The listing builds one solid part. Answer for the finished solid, in the listing's coordinates (mm). A direction names the side the tool comes from. Coordinates: 2 decimals unless noted, no trailing zeros. Order: outer loops, then holes, each group sorted by start corner. A loop starts at its lowest first (then second) coordinate and runs counter-clockwise, first axis right, second up. Notation, with made-up numbers: (-37.5, 12.25) -> (18.5, 12.25) arc R10 ccw to (18.5, 21.25) -> close; hole circle Ø2 at (-21.5, 35.25). An arc over 180 degrees is marked (long way). Return JSON: item names as keys, results as strings.
```python
from build123d import *

# Parameters (mm, degrees)
EXTRUDE_1_DEPTH     = 8.5
SKETCH_2_R          = 1.7
CUT_EXTRUDE_1_DEPTH = 34.737960816


with BuildPart() as part:
    # 草图1 → 凸台-拉伸1 (new body)
    with BuildSketch(Plane(origin=(0, 0, 0), x_dir=(1, 0, 0), z_dir=(0, 1, 0))):
        with BuildLine():
            Line((-25, -21), (25, -21))
            Line((25, -21), (25, -9))
            Line((25, -9), (11.788272368, -9))
            Line((11.788272368, -9), (6.375, -11.899973739))
            ThreePointArc((6.375, -11.899973739), (0, -13.5), (-6.375, -11.899973739))
            Line((-6.375, -11.899973739), (-11.788272368, -9))
            Line((-11.788272368, -9), (-25, -9))
            Line((-25, -9), (-25, -21))
        make_face()
    extrude(amount=EXTRUDE_1_DEPTH)

    # 草图2 → 切除-拉伸1 (cut, through all)
    with BuildSketch(Plane(origin=(0, 8.5, 0), x_dir=(1, 0, 0), z_dir=(0, 1, 0))):
        with Locations(Location((6, -17, 0), (0, 0, 270))):
            Circle(SKETCH_2_R)
        with Locations(Location((-6, -17, 0), (0, 0, 90))):
            Circle(SKETCH_2_R)
    extrude(amount=-CUT_EXTRUDE_1_DEPTH, mode=Mode.SUBTRACT)


solid = part.part
```
Item 1: The part is cut by section A-A on z = 17. Determine the outline of the cut face in (x, y), plus the area to 3 significant figures.
Answer list:
{"outline": "(-25, 0) -> (-7.7, 0) -> (-7.7, 8.5) -> (-25, 8.5) -> close; (-4.3, 0) -> (4.3, 0) -> (4.3, 8.5) -> (-4.3, 8.5) -> close; (7.7, 0) -> (25, 0) -> (25, 8.5) -> (7.7, 8.5) -> close", "area": "367 mm2"}
Item 2: The part is cut by section D-D on z = 10. Determine the outline of the cut face in (x, y).
Answer list:
{"outline": "(-25, 0) -> (-9.92, 0) -> (-9.92, 8.5) -> (-25, 8.5) -> close; (9.92, 0) -> (25, 0) -> (25, 8.5) -> (9.92, 8.5) -> close"}
Item 3: The part is cut by section C-C on x = 5.5. Determine the outline of the cut face in (y, z), plus the area to 3 significant figures.
Answer list:
{"outline": "(0, 12.33) -> (8.5, 12.33) -> (8.5, 15.38) -> (0, 15.38) -> close; (0, 18.62) -> (8.5, 18.62) -> (8.5, 21) -> (0, 21) -> close", "area": "46.1 mm2"}
Item 4: Find the intervals of material crossed by probe 1 along X at (y, z) = (3, 17); probe 2 along X at (y, z) = (7.25, 18); probe 3 along Z at (x, y) = (-6, 4), in increasing order.
Answer list:
{"probe 1": "-25 to -7.7, -4.3 to 4.3, 7.7 to 25", "probe 2": "-25 to -7.37, -4.63 to 4.63, 7.37 to 25", "probe 3": "12.09 to 15.3, 18.7 to 21"}
Item 5: Flat-ended cylindrical pins translate along their axes: pin 1 (2 mm diameter, centred on x = -7.5, z = 10.5, fed in from -Y); pin 2 (3 mm diameter, centred on x = -6, z = 17, fed in from -Y). Find the tip coordinate at first contact, or state that the pin passes through.
Answer list:
{"pin 1": "y = 0", "pin 2": "through"}
Item 6: Determine the mould class of faces 3 (the flat face through (18, 4, 9)), 4 (the cylindrical face through (0.1, 4.2, 13.5)), 5 (the flat face through (-25, 4, 15)) for opening direction X: pulls with the +X half, pulls with the -X half, needs draft (parallel to the pull), parting line crosses it, or undercut.
Answer list:
{"face 3": "needs draft", "face 4": "undercut", "face 5": "pulls with the -X half"}
Item 7: Which of the six approach directions +Z, -Z, +X, -X, +Y, -Y give full straight-line access (tool end or side, diameter ignored) to faces 1 (the cylindrical face through (5.35, 4.31, 18.57)), 2 (the flat face through (9.12, 4.19, 10.43))?
Answer list:
{"face 1": "+Y, -Y", "face 2": "-Z, +Y, -Y"}
Item 8: The part is cut by section B-B on y = 7. Determine the outline of the cut face in (x, z) (3 decimals), plus the area to 3 significant figures.
Answer list:
{"outline": "(-25, 9) -> (-11.788, 9) -> (-6.375, 11.9) arc R13.5 cw to (6.375, 11.9) -> (11.788, 9) -> (25, 9) -> (25, 21) -> (-25, 21) -> close; hole circle Ø3.4 at (-6, 17); hole circle Ø3.4 at (6, 17)", "area": "515 mm2"}
